```python
from build123d import *

# Parameters (mm, degrees)
SKETCH7_W                                           = 122
SKETCH7_H                                           = 45
BOSS_EXTRUDE1_DEPTH                                 = 10
SKETCH9_R                                           = 2.5
BOSS_EXTRUDE2_DEPTH                                 = 10
BOSS_EXTRUDE3_START                                 = -25
SKETCH10_R                                          = 40
BOSS_EXTRUDE3_DEPTH                                 = 25
SKETCH11_R                                          = 2.5
CUT_EXTRUDE5_DEPTH                                  = 97.15612305
CUT_EXTRUDE6_DEPTH                                  = 95.053176448
CBORE_FOR_4_BINDING_HEAD_MACHINE_SCREW1_D           = 3.2639
CBORE_FOR_4_BINDING_HEAD_MACHINE_SCREW1_CBORE_D     = 6.74624
CBORE_FOR_4_BINDING_HEAD_MACHINE_SCREW1_CBORE_DEPTH = 1.7272


with BuildPart() as part:
    # Sketch7 → Boss-Extrude1 (new body)
    with BuildSketch(Plane(origin=(0, 0, 0), x_dir=(1, 0, 0), z_dir=(0, 1, 0))):
        with Locations((0, 22.5)):
            Rectangle(SKETCH7_W, SKETCH7_H)
    extrude(amount=BOSS_EXTRUDE1_DEPTH)

    # Sketch9 → Boss-Extrude2 (add)
    # profile 1 of 9: a face of its own
    with BuildSketch(Plane(origin=(0, 10, 0), x_dir=(1, 0, 0), z_dir=(0, 1, 0))):
        with BuildLine():
            ThreePointArc((35.858512086, 0), (40.682190705, 10.793495465), (42.333, 22.5))
            ThreePointArc((42.333, 22.5), (40.682190705, 34.206504535), (35.858512086, 45))
            Line((35.858512086, 45), (-35.858512086, 45))
            ThreePointArc((-35.858512086, 45), (-42.333, 22.5), (-35.858512086, 0))
            Line((-35.858512086, 0), (35.858512086, 0))
        make_face()
        with Locations((37.333, 22.5)):
            Circle(SKETCH9_R, mode=Mode.SUBTRACT)
        with Locations((-37.333, 22.5)):
            Circle(SKETCH9_R, mode=Mode.SUBTRACT)
    # profile 2 of 9: a face of its own
    with BuildSketch(Plane(origin=(0, 10, 0), x_dir=(1, 0, 0), z_dir=(0, 1, 0))):
        with Locations((37.333, 22.5)):
            Circle(SKETCH9_R)
    # profile 3 of 9: a face of its own
    with BuildSketch(Plane(origin=(0, 10, 0), x_dir=(1, 0, 0), z_dir=(0, 1, 0))):
        with Locations((-37.333, 22.5)):
            Circle(SKETCH9_R)
    # profile 4 of 9: a face of its own
    with BuildSketch(Plane(origin=(0, 10, 0), x_dir=(1, 0, 0), z_dir=(0, 1, 0))):
        with BuildLine():
            ThreePointArc((-35.858512086, 0), (0, -19.833), (35.858512086, 0))
            Line((35.858512086, 0), (-35.858512086, 0))
        make_face()
        with Locations((-18.6665, -9.831326399)):
            Circle(SKETCH9_R, mode=Mode.SUBTRACT)
        with Locations((18.6665, -9.831326399)):
            Circle(SKETCH9_R, mode=Mode.SUBTRACT)
    # profile 5 of 9: a face of its own
    with BuildSketch(Plane(origin=(0, 10, 0), x_dir=(1, 0, 0), z_dir=(0, 1, 0))):
        with Locations((18.6665, -9.831326399)):
            Circle(SKETCH9_R)
    # profile 6 of 9: a face of its own
    with BuildSketch(Plane(origin=(0, 10, 0), x_dir=(1, 0, 0), z_dir=(0, 1, 0))):
        with Locations((-18.6665, -9.831326399)):
            Circle(SKETCH9_R)
    # profile 7 of 9: a face of its own
    with BuildSketch(Plane(origin=(0, 10, 0), x_dir=(1, 0, 0), z_dir=(0, 1, 0))):
        with BuildLine():
            Line((-35.858512086, 45), (35.858512086, 45))
            ThreePointArc((35.858512086, 45), (0, 64.833), (-35.858512086, 45))
        make_face()
        with Locations((-18.6665, 54.831326399)):
            Circle(SKETCH9_R, mode=Mode.SUBTRACT)
        with Locations((18.6665, 54.831326399)):
            Circle(SKETCH9_R, mode=Mode.SUBTRACT)
    # profile 8 of 9: a face of its own
    with BuildSketch(Plane(origin=(0, 10, 0), x_dir=(1, 0, 0), z_dir=(0, 1, 0))):
        with Locations((18.6665, 54.831326399)):
            Circle(SKETCH9_R)
    # profile 9 of 9: a face of its own
    with BuildSketch(Plane(origin=(0, 10, 0), x_dir=(1, 0, 0), z_dir=(0, 1, 0))):
        with Locations((-18.6665, 54.831326399)):
            Circle(SKETCH9_R)
    extrude(amount=-BOSS_EXTRUDE2_DEPTH)

    # Sketch10 → Boss-Extrude3 (add)
    # profile 1 of 3: a face of its own
    with BuildSketch(Plane.XZ.offset(BOSS_EXTRUDE3_START)):
        with BuildLine():
            ThreePointArc((-41.833001327, -45), (0, -70), (41.833001327, -45))
            Line((41.833001327, -45), (35.858512086, -45))
            ThreePointArc((35.858512086, -45), (0, -64.833), (-35.858512086, -45))
            Line((-35.858512086, -45), (-41.833001327, -45))
        make_face()
    # profile 2 of 3: a face of its own
    with BuildSketch(Plane.XZ.offset(BOSS_EXTRUDE3_START)):
        with BuildLine():
            ThreePointArc((41.833001327, -45), (46.061467427, -34.101345547), (47.5, -22.5))
            ThreePointArc((47.5, -22.5), (46.061467427, -10.898654453), (41.833001327, 0))
            Line((41.833001327, 0), (35.858512086, 0))
            ThreePointArc((35.858512086, 0), (0, 19.833), (-35.858512086, 0))
            Line((-35.858512086, 0), (-41.833001327, 0))
            ThreePointArc((-41.833001327, 0), (-47.5, -22.5), (-41.833001327, -45))
            Line((-41.833001327, -45), (-35.858512086, -45))
            ThreePointArc((-35.858512086, -45), (0, -64.833), (35.858512086, -45))
            Line((35.858512086, -45), (41.833001327, -45))
        make_face()
        with Locations(Location((0, -22.5, 0), (0, 0, 270))):
            Circle(SKETCH10_R, mode=Mode.SUBTRACT)
    # profile 3 of 3: a face of its own
    with BuildSketch(Plane.XZ.offset(BOSS_EXTRUDE3_START)):
        with BuildLine():
            Line((35.858512086, 0), (41.833001327, 0))
            ThreePointArc((41.833001327, 0), (0, 25), (-41.833001327, 0))
            Line((-41.833001327, 0), (-35.858512086, 0))
            ThreePointArc((-35.858512086, 0), (0, 19.833), (35.858512086, 0))
        make_face()
    extrude(amount=BOSS_EXTRUDE3_DEPTH)

    # Sketch11 → Cut-Extrude5 (cut, through all)
    with BuildSketch(Plane.XY):
        with Locations((-53.5, 5)):
            Circle(SKETCH11_R)
        with Locations((53.5, 5)):
            Circle(SKETCH11_R)
    extrude(amount=-CUT_EXTRUDE5_DEPTH, mode=Mode.SUBTRACT)

    # Sketch12 → Cut-Extrude6 (cut, through all)
    with BuildSketch(Plane(origin=(0, 10, 0), x_dir=(1, 0, 0), z_dir=(0, 1, 0))):
        with BuildLine():
            Line((-17.78, 58.331154042), (-17.78, 66.546811462))
            ThreePointArc((-17.78, 66.546811462), (0, 70), (17.78, 66.546811462))
            Line((17.78, 66.546811462), (17.78, 58.331154042))
            ThreePointArc((17.78, 58.331154042), (0, 62.5), (-17.78, 58.331154042))
        make_face()
    extrude(amount=CUT_EXTRUDE6_DEPTH, mode=Mode.SUBTRACT)

    # CBORE for #4 Binding Head Machine Screw1 (through all)
    with Locations(Plane.XZ):
        with Locations((-18.6665, 9.831326399), (18.6665, 9.831326399), (37.333, -22.5), (18.6665, -54.831326399), (-18.6665, -54.831326399), (-37.333, -22.5)):
            CounterBoreHole(CBORE_FOR_4_BINDING_HEAD_MACHINE_SCREW1_D / 2, CBORE_FOR_4_BINDING_HEAD_MACHINE_SCREW1_CBORE_D / 2, CBORE_FOR_4_BINDING_HEAD_MACHINE_SCREW1_CBORE_DEPTH)


solid = part.part
```
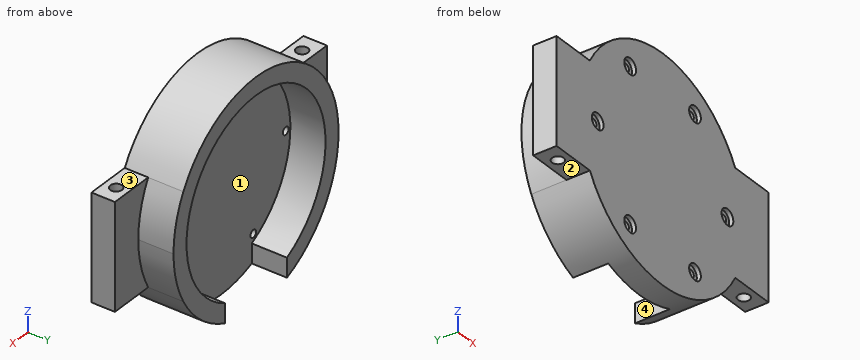
Design review of the part built by this model. Coordinates are the model's own, in mm. Face numbers are marked on the shaded views. A direction names the side the tool comes from. Give positions to 0.01 mm unless a question says otherwise; leave off trailing zeros. Write each loop counter-clockwise with the first axis right and the second up, starting at its lowest first coordinate (ties: lowest second). Pieces come first, ordered by that corner, then holes. Notation, with made-up numbers: (80.25, 16.25) - (96.25, 16.25) arc R20 cw to (96.25, 52.25) - close; hole circle Ø1 at (-4.5, 5.5). An arc over 180 degrees is marked (long way). Return JSON: item names as keys, results as strings. Group by question number.
(1) We need section B-B, the plane y = 19.25. Give the boundary of the cut face in (x, z), then the cut area to 3 significant figures.
(2) To check wall thickness, follow probe 1 along X at (y, z) = (17.25, -22.5); probe 2 along X at (y, z) = (6.5, -17.5); probe 3 along X at (y, z) = (4.25, -26). State the ranges of each line that lie inside material, in increasing order.
(3) We need section D-D, the plane x = 0. Give the boundary of the cut face in (y, z), then the cut area to 3 significant figures.
(4) We need section A-A, the plane x = -53.5. Give the boundary of the cut face in (y, z).
(5) Machinability: for the marked faces 1, 2, 3 and 4, which of the approach directions +Z, -Z, +X, -X, +Y, -Y give a long, thin tool a straight path to every point of the face, cutting with its end or side? Answer none if there is none.
(6) We need section C-C, the plane y = 5. Give the number of separate pieces and of enclosed holes in the cut face, then the cut area to 3 significant figures.
(7) Insertion check: pin 1 (9.5 mm diameter, centred on x = 50, z = -11.5, fed in from +Y); pin 2 (1 mm diameter, centred on y = 14.5, z = -42, fed in from +X); pin 3 (12 mm diameter, centred on x = 13.5, y = 21.5, fed in from +Z); pin 4 (6 mm diameter, centred on x = -47, z = -45, fed in from +Y). Each pin has a flat end and moves straight along its axis. Give the tip position at first contact, or say it passes through.
Reported:
{
 "1": {"outline": "(-17.78, -66.55) - (-17.78, -58.33) arc R40 cw (long way) to (17.78, -58.33) - (17.78, -66.55) arc R47.5 ccw (long way) to start", "area": "1,790 mm2"},
 "2": {"probe 1": "x = -47.5 to -40, 40 to 47.5", "probe 2": "x = -61 to -55.5, -51.5 to 51.5, 55.5 to 61", "probe 3": "x = -61 to -55.88, -51.12 to 51.12, 55.88 to 61"},
 "3": {"outline": "(0, -70) - (10, -70) - (10, 17.5) - (25, 17.5) - (25, 25) - (0, 25) - close", "area": "1,060 mm2"},
 "4": {"outline": "(0, -45) - (2.5, -45) - (2.5, 0) - (0, 0) - close; (7.5, -45) - (10, -45) - (10, 0) - (7.5, 0) - close"},
 "5": {"face 1": "+Y", "face 2": "-Z, -X, +Y, -Y", "face 3": "+Z, +X, +Y, -Y", "face 4": "-Z, +Y"},
 "6": {"separate pieces": "3", "enclosed holes": "6", "area": "7,970 mm2"},
 "7": {"pin 1": "stops at y = 25", "pin 2": "stops at x = 43.53", "pin 3": "stops at z = 24.4", "pin 4": "stops at y = 10"}
}
